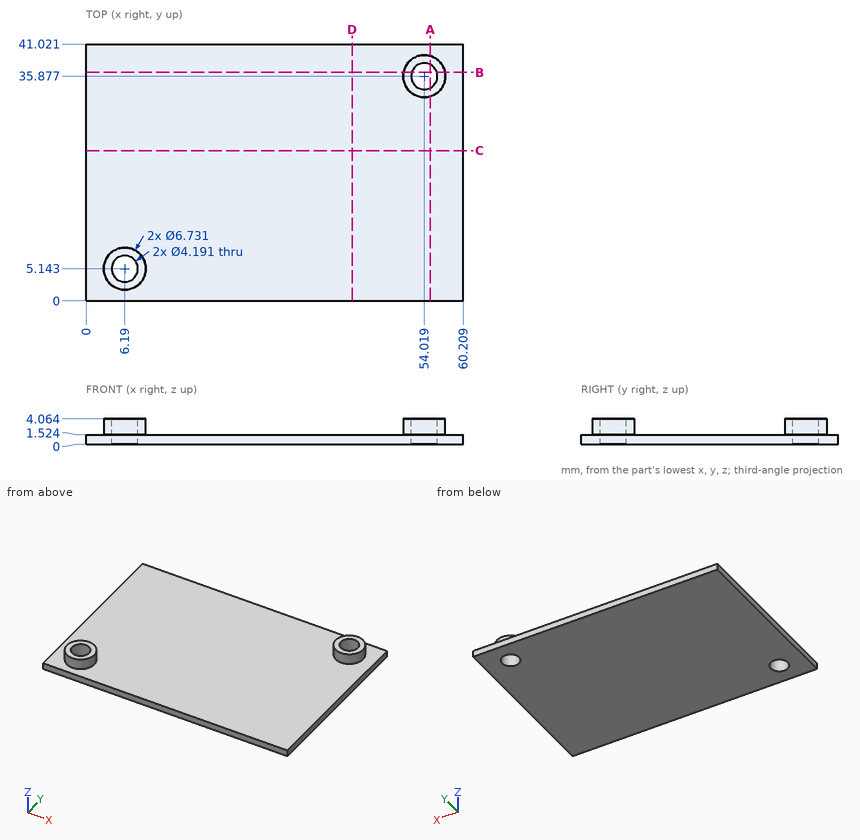
Verification items for this drawing (mm, ordinates from the low corner). Give positions to 0.01 mm unless a question says otherwise; leave off trailing zeros. Loops run counter-clockwise (first coordinate to the right, second up) from the corner with the lowest first, then second, coordinate; pieces in that order, holes last. Notation, with made-up numbers: M -3,1.5 L 20,1.5 A19 cw 20,11.5 Z; hole C 66,20 d11. An arc over 180 degrees is marked long. Return JSON: item names as keys, results as strings. Group by question number.
1. Go/stop test with flat-tipped pins: pin 1 (12.5 mm diameter, centred on x = 39.5, y = 30.5, fed in from +Z); pin 2 (1.5 mm diameter, centred on y = 8.5, z = 3.5, fed in from -X). Record where each tip stops, or that it passes through.
2. Cross-section at D-D on x = 42.5. Record the boundary of the cut face in (y, z) (1 decimal).
3. Cross-section at B-B on y = 36.5. Record the boundary of the cut face in (x, z) (1 decimal).
4. Cross-section at C-C on y = 24. Record the boundary of the cut face in (x, z) (1 decimal).
5. Cross-section at A-A on x = 55. Record the boundary of the cut face in (y, z) (1 decimal).
6. Thickness scan on L1, parallel to Z at x = 42, y = 4 (1 decimal); L2, parallel to X at y = 6, z = 1.3; L3, parallel to Y at x = 4.5, z = 0.9 (1 decimal). Record the ranges inside material, lowest first.
Return value:
{
 "1": {"pin 1": "z = 1.52", "pin 2": "x = 4.06"},
 "2": {"outline": "M 0,0 L 41,0 L 41,1.5 L 0,1.5 Z"},
 "3": {"outline": "M 0,0 L 52,0 L 52,4.1 L 50.7,4.1 L 50.7,1.5 L 0,1.5 Z; M 56,0 L 60.2,0 L 60.2,1.5 L 57.3,1.5 L 57.3,4.1 L 56,4.1 Z"},
 "4": {"outline": "M 0,0 L 60.2,0 L 60.2,1.5 L 0,1.5 Z"},
 "5": {"outline": "M 0,0 L 34,0 L 34,4.1 L 32.7,4.1 L 32.7,1.5 L 0,1.5 Z; M 37.7,0 L 41,0 L 41,1.5 L 39.1,1.5 L 39.1,4.1 L 37.7,4.1 Z"},
 "6": {"L1": "0 to 1.5", "L2": "0 to 4.28, 8.1 to 60.21", "L3": "0 to 3.9, 6.4 to 41"}
}
